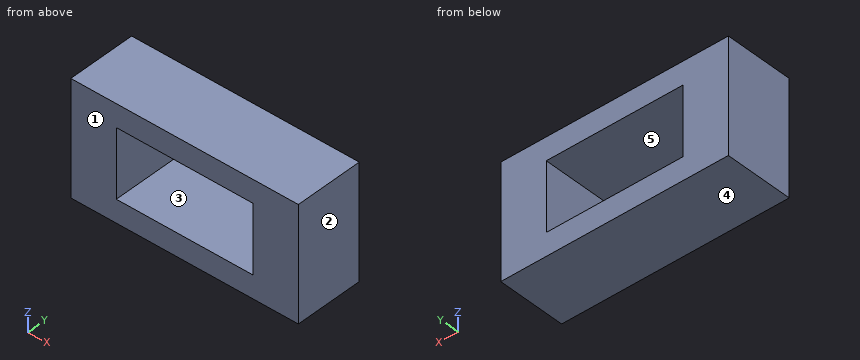
```python
from build123d import *

# Parameters (mm, degrees)
F0_W     = 76.2
F0_H     = 38.1
F1_DEPTH = 38.1


with BuildPart() as f1:
    # F0 (on Front) → F1 (new body)
    with BuildSketch(Plane.XZ):
        Polygon((-53.589837, -26.378524), (-53.589837, -39.078524), (-28.189837, -39.078524), (48.010163, -39.078524), (73.410163, -39.078524), (73.410163, -26.378524), (73.410163, 11.721476), (73.410163, 24.421476), (48.010163, 24.421476), (-28.189837, 24.421476), (-53.589837, 24.421476), (-53.589837, 11.721476), align=None)
        with Locations((9.910163, -7.328524)):
            Rectangle(F0_W, F0_H, mode=Mode.SUBTRACT)
    extrude(amount=F1_DEPTH)


solid = f1.part
```
Geometry: final body of the model. Coordinates: model frame, mm. Face numbers are marked on the shaded views. A direction names the side the tool comes from. Coordinates: 2 decimals unless noted, no trailing zeros. Order: outer loops, then holes, each group sorted by start corner. A loop starts at its lowest first (then second) coordinate and runs counter-clockwise, first axis right, second up. Notation, with made-up numbers: (-24, -29) -> (-17, -29) arc R12 ccw to (-17, -23) -> close; hole circle Ø5 at (-24, 68). An arc over 180 degrees is marked (long way). Answer in a Markdown table with one row per item.
Item 1: Section B-B on z = -23.5. Output: boundary loops of the cut face in (x, y).
Return value:
| item | result |
|---|---|
| outline | (-53.59, -38.1) -> (-28.19, -38.1) -> (-28.19, 0) -> (-53.59, 0) -> close; (48.01, -38.1) -> (73.41, -38.1) -> (73.41, 0) -> (48.01, 0) -> close |
Item 2: Section C-C on y = -11.5. Output: boundary loops of the cut face in (x, z), plus the area to 3 significant figures.
Return value:
| item | result |
|---|---|
| outline | (-53.59, -39.08) -> (73.41, -39.08) -> (73.41, 24.42) -> (-53.59, 24.42) -> close; hole (-28.19, -26.38) -> (48.01, -26.38) -> (48.01, 11.72) -> (-28.19, 11.72) -> close |
| area | 5,160 mm² |
Item 3: Section A-A on x = -10.5. Output: boundary loops of the cut face in (y, z).
Return value:
| item | result |
|---|---|
| outline | (-38.1, -39.08) -> (0, -39.08) -> (0, -26.38) -> (-38.1, -26.38) -> close; (-38.1, 11.72) -> (0, 11.72) -> (0, 24.42) -> (-38.1, 24.42) -> close |
Item 4: Draft query along X for the marked faces 1, 2 and 3. Return one class per face: released by +X, released by -X, zero draft, split by the parting line, or undercut.
Return value:
| item | result |
|---|---|
| face 1 | zero draft |
| face 2 | released by +X |
| face 3 | undercut |
Item 5: Access query for the marked faces 4 and 5. Directions: +Z, -Z, +X, -X, +Y, -Y. A direction counts if a zero-diameter tool reaches every point of the face in a straight line with its end or side. Return the directions, or none.
Return value:
| item | result |
|---|---|
| face 4 | -Z, +X, -X, +Y, -Y |
| face 5 | +Y, -Y |
Item 6: Ray query, L1, parallel to Z at x = -24, y = -18; L2, parallel to X at y = -31.5, z = -8.5. Return the intervals inside material, ascending.
Return value:
| item | result |
|---|---|
| L1 | z = -39.08 to -26.38, 11.72 to 24.42 |
| L2 | x = -53.59 to -28.19, 48.01 to 73.41 |
